CAD build for the part. Positions are in the model's coordinates, mm. A direction names the side the tool comes from. Give positions to 0.01 mm unless a question says otherwise; leave off trailing zeros. Order: outer loops, then holes, each group sorted by start corner. A loop starts at its lowest first (then second) coordinate and runs counter-clockwise, first axis right, second up.
Item 1: Two-plate mould, pull along Y, no slides. Class faces 5 (the flat face through (-11.45, -11.67, 10.4)), 6 (the cylindrical face through (0.605, -10.48, 0.989)), 7 (the flat face through (-11.17, 12.13, 0.96)): released by +Y, released by -Y, zero draft, split by the parting line, or undercut.
Item 2: Flat gauge pins, fed straight in: P1, Ø7.5, axis at y = -3.5, z = 10.5, coming from the +X side; P2, Ø0.9, axis at x = 11.5, y = 17, coming from the -Z side; P3, Ø6, axis at x = -9, z = 3, coming from the +Y side; P4, Ø6, axis at y = -4, z = 11, coming from the -X side. Where does each tip first touch, or does it go through?
Item 3: Wall check: L1, parallel to X at y = 7, z = 14; L2, parallel to X at y = 10, z = 9.25; L3, parallel to Y at x = 3, z = 1. Give the ranges that are in metal, low to high.
Item 4: Which spindle directions (+Z, -Z, +X, -X, +Y, -Y) get a long thin tool onto all of the face, cutting with end or side? Do faces 1 (the flat face through (-12.07, 7, 8)), 2 (the flat face through (0, -8, 1.95)), 3 (the cylindrical face through (-0.143, 5.981, 1.394)), 4 (the flat face through (-4, -15.948, 1)). Say none if no direction does.
Item 5: Band-saw the part on A-A on z = 2.5. Give the cut face in (x, y).
Item 6: Band-saw the part on B-B on x = -4. Give the cut face in (y, z).
Item 7: Band-saw the part on C-C on y = -2. Give the cut face in (x, z), plus the area to 3 significant figures.
Item 8: Band-saw the part on D-D on z = 11.5. Give the cut face in (x, y), plus the area to 3 significant figures.
```python
from build123d import *

# Parameters (mm, degrees)
BOSS_EXTRUDE1_DEPTH = 3.67
SKETCH2_W           = 3.67
SKETCH2_H           = 9.687937517
BOSS_EXTRUDE2_DEPTH = 9.735
SKETCH3_W           = 3.67
SKETCH3_H           = 26.515
BOSS_EXTRUDE3_DEPTH = 5.622062483
BOSS_EXTRUDE4_DEPTH = 20.5
SKETCH5_W           = 3.67
SKETCH5_H           = 15.31
BOSS_EXTRUDE5_DEPTH = 13.38
BOSS_EXTRUDE6_DEPTH = 2.35
SKETCH7_W           = 1.85
SKETCH7_H           = 17.78
CUT_EXTRUDE1_DEPTH  = 16.310000003
CUT_EXTRUDE2_REACH  = 27.99
SKETCH9_W           = 1.85
SKETCH9_H           = 17.78
CUT_EXTRUDE3_DEPTH  = 16.310000003
CUT_EXTRUDE4_REACH  = 26.67
CUT_EXTRUDE5_REACH  = 26.67
CUT_EXTRUDE6_DEPTH  = 26.99
CUT_EXTRUDE7_DEPTH  = 2.95
SKETCH15_W          = 1.68
SKETCH15_H          = 2.795
SKETCH16_W          = 1.68
SKETCH16_H          = 2.795
FILLET1_R           = 0.2
CUT_EXTRUDE8_DEPTH  = 1.31


with BuildPart() as part:
    # Sketch1 → Boss-Extrude1 (new body)
    with BuildSketch(Plane(origin=(-13.92, 0, 0), x_dir=(0, -1, 0), z_dir=(-1, 0, 0))):
        Polygon((19.9475, 5.622062483), (3.1675, 15.31), (3.1675, 5.622062483), align=None)
    extrude(amount=-BOSS_EXTRUDE1_DEPTH)

    # Sketch2 → Boss-Extrude2 (add)
    with BuildSketch(Plane(origin=(0, -3.1675, 0), x_dir=(-1, 0, 0), z_dir=(0, 1, 0))):
        with Locations((12.085, 10.466031242)):
            Rectangle(SKETCH2_W, SKETCH2_H)
    extrude(amount=BOSS_EXTRUDE2_DEPTH)

    # Sketch3 → Boss-Extrude3 (add)
    with BuildSketch(Plane(origin=(0, 0, 5.622062483), x_dir=(-1, 0, 0), z_dir=(0, 0, -1))):
        with Locations((12.085, -6.69)):
            Rectangle(SKETCH3_W, SKETCH3_H)
    extrude(amount=BOSS_EXTRUDE3_DEPTH)

    # Sketch4 → Boss-Extrude4 (add)
    with BuildSketch(Plane(origin=(-10.25, 0, 0), x_dir=(0, 0, -1), z_dir=(1, 0, 0))):
        with BuildLine():
            Line((3e-09, -19.9475), (-1.949999997, -19.9475))
            Line((-1.949999997, -19.9475), (-1.949999997, 4.6175))
            ThreePointArc((-1.949999997, 4.6175), (-1.37885822, 5.996358223), (3e-09, 6.5675))
            Line((3e-09, 6.5675), (3e-09, -19.9475))
        make_face()
    extrude(amount=BOSS_EXTRUDE4_DEPTH)

    # Sketch5 → Boss-Extrude5 (add)
    with BuildSketch(Plane(origin=(0, 6.5675, 0), x_dir=(-1, 0, 0), z_dir=(0, 1, 0))):
        with Locations((12.085, 7.655)):
            Rectangle(SKETCH5_W, SKETCH5_H)
    extrude(amount=BOSS_EXTRUDE5_DEPTH)

    # Sketch6 → Boss-Extrude6 (add)
    with BuildSketch(Plane(origin=(10.25, 0, 0), x_dir=(0, 0, -1), z_dir=(1, 0, 0))):
        Polygon((-15.31, -3.1675), (-15.31, 19.9475), (2e-09, 19.9475), (2e-09, -19.947499999), (-5.622062484, -19.947499999), align=None)
    extrude(amount=BOSS_EXTRUDE6_DEPTH)

    # Sketch7 → Cut-Extrude1 (cut, through all)
    with BuildSketch(Plane.XY.offset(15.31)):
        with Locations((12.995, 11.0575)):
            Rectangle(SKETCH7_W, SKETCH7_H)
    extrude(amount=-CUT_EXTRUDE1_DEPTH, mode=Mode.SUBTRACT)

    # Sketch8 → Cut-Extrude2 (cut, up to next)
    with BuildSketch(Plane(origin=(12.07, 0, 0), x_dir=(0, 0, -1), z_dir=(1, 0, 0)), mode=Mode.PRIVATE) as cut_extrude2_sk1:
        with BuildLine():
            Line((-8.04306505, 17.864239052), (-5.959804102, 19.9475))
            Line((-5.959804102, 19.9475), (-15.31, 19.9475))
            Line((-15.31, 19.9475), (-15.31, 10.26298277))
            ThreePointArc((-15.31, 10.26298277), (-13.200981436, 15.521010933), (-8.04306505, 17.864239052))
        make_face()
    cut_extrude2_tool1 = extrude(cut_extrude2_sk1.sketch, amount=-CUT_EXTRUDE2_REACH, mode=Mode.PRIVATE) & part.part
    add(cut_extrude2_tool1.solids().sort_by_distance((12.07, 17.788809, 12.169828))[0], mode=Mode.SUBTRACT)

    # Sketch9 → Cut-Extrude3 (cut, through all)
    with BuildSketch(Plane.XY.offset(15.31)):
        with Locations((-12.995, 11.0575)):
            Rectangle(SKETCH9_W, SKETCH9_H)
    extrude(amount=-CUT_EXTRUDE3_DEPTH, mode=Mode.SUBTRACT)

    # Sketch10 → Cut-Extrude4 (cut, up to next)
    with BuildSketch(Plane.ZY.offset(12.07), mode=Mode.PRIVATE) as cut_extrude4_sk1:
        Polygon((1.95, 13.1175), (1.95, 19.9475), (0, 19.9475), (0, 11.1675), align=None)
    cut_extrude4_tool1 = extrude(cut_extrude4_sk1.sketch, amount=-CUT_EXTRUDE4_REACH, mode=Mode.PRIVATE) & part.part
    add(cut_extrude4_tool1.solids().sort_by_distance((-12.07, 16.024701, 0.934401))[0], mode=Mode.SUBTRACT)

    # Sketch11 → Cut-Extrude5 (cut, up to next)
    with BuildSketch(Plane.ZY.offset(12.07), mode=Mode.PRIVATE) as cut_extrude5_sk1:
        with BuildLine():
            Line((5.959804102, 19.9475), (8.04306505, 17.864239052))
            ThreePointArc((8.04306505, 17.864239052), (13.200981436, 15.521010933), (15.31, 10.26298277))
            Line((15.31, 10.26298277), (15.31, 19.9475))
            Line((15.31, 19.9475), (5.959804102, 19.9475))
        make_face()
    cut_extrude5_tool1 = extrude(cut_extrude5_sk1.sketch, amount=-CUT_EXTRUDE5_REACH, mode=Mode.PRIVATE) & part.part
    add(cut_extrude5_tool1.solids().sort_by_distance((-12.07, 17.788809, 12.169828))[0], mode=Mode.SUBTRACT)

    # Sketch12 → Cut-Extrude6 (cut, through all)
    with BuildSketch(Plane(origin=(12.07, 0, 0), x_dir=(0, 0, -1), z_dir=(1, 0, 0))):
        Polygon((-1.95, 19.9475), (-1.95, 13.1175), (0, 11.1675), (0, 19.9475), align=None)
    extrude(amount=-CUT_EXTRUDE6_DEPTH, mode=Mode.SUBTRACT)

    # Sketch13 → Cut-Extrude7 (cut, through all)
    with BuildSketch(Plane.XY.offset(1.949999997)):
        with BuildLine():
            Line((-6.395488685, -12.9475), (-2.104511315, -12.9475))
            ThreePointArc((-2.104511315, -12.9475), (-0.604511315, -14.4475), (-2.104511315, -15.9475))
            Line((-2.104511315, -15.9475), (-6.395488685, -15.9475))
            ThreePointArc((-6.395488685, -15.9475), (-7.895488685, -14.4475), (-6.395488685, -12.9475))
        make_face()
        with BuildLine():
            Line((2.104511315, -8.947499999), (6.395488685, -8.947499999))
            ThreePointArc((6.395488685, -8.947499999), (7.895488685, -10.447499999), (6.395488685, -11.947499999))
            Line((6.395488685, -11.947499999), (2.104511315, -11.947499999))
            ThreePointArc((2.104511315, -11.947499999), (0.604511315, -10.447499999), (2.104511315, -8.947499999))
        make_face()
    extrude(amount=-CUT_EXTRUDE7_DEPTH, mode=Mode.SUBTRACT)

    # Sketch15 → Revolve1 (revolve)
    with BuildSketch(Plane.XY.offset(7.655)):
        with Locations((12.91, 11.61)):
            Rectangle(SKETCH15_W, SKETCH15_H)
    revolve(axis=Axis((12.07, 10.2125, 7.655), (1, 0, 0)))

    # Sketch16 → Revolve2 (revolve)
    with BuildSketch(Plane.XY.offset(7.655)):
        with Locations((-12.91, 11.61)):
            Rectangle(SKETCH16_W, SKETCH16_H)
    revolve(axis=Axis((-13.75, 10.2125, 7.655), (1, 0, 0)))

    # Fillet1
    fillet1_edges = [part.edges().sort_by_distance(p)[0] for p in [
        (13.75, 7.4175, 7.655),
        (-13.75, 7.4175, 7.655),
    ]]
    fillet(fillet1_edges, radius=FILLET1_R)

    # Sketch17 → Cut-Extrude8 (cut)
    with BuildSketch(Plane(origin=(-13.92, -19.9475, 5.622062483), x_dir=(0, 0, 1), z_dir=(-1, 0, 0))):
        Polygon((9.687937517, 22.115), (-5.622062486, 22.115), (-5.622062483, 0), (0, 0), (9.687937517, 16.78), align=None)
    extrude(amount=-CUT_EXTRUDE8_DEPTH, mode=Mode.SUBTRACT)


solid = part.part
```
The answers:
1. face 5: released by -Y
1. face 6: undercut
1. face 7: released by +Y
2. P1: stops at x = 12.6
2. P2: stops at z = 1.95
2. P3: stops at y = 19.95
2. P4: stops at x = -12.61
3. L1: x = -12.07 to -10.25, 10.25 to 12.07
3. L2: x = -13.75 to -10.25, 10.25 to 13.75
3. L3: y = -19.95 to -11.95, -8.95 to 6.29
4. face 1: -X
4. face 2: +Z, +Y, -Y
4. face 3: +Z, +Y
4. face 4: +Z, -Z
5. outline: (-12.61, -19.95) - (-10.25, -19.95) - (-10.25, 19.95) - (-12.07, 19.95) - (-12.07, 2.17) - (-12.61, 2.17) - close; (10.25, -19.95) - (12.6, -19.95) - (12.6, 2.17) - (12.07, 2.17) - (12.07, 19.95) - (10.25, 19.95) - close
6. outline: (-19.95, 0) - (-15.95, 0) - (-15.95, 1.95) - (-19.95, 1.95) - close; (-12.95, 0) - (6.57, 0) arc R1.95 ccw to (4.62, 1.95) - (-12.95, 1.95) - close
7. outline: (-12.61, 0) - (12.6, 0) - (12.6, 15.31) - (10.25, 15.31) - (10.25, 1.95) - (-10.25, 1.95) - (-10.25, 15.31) - (-12.61, 15.31) - close
7. area: 112 mm2
8. outline: (-12.61, -9.77) - (-10.25, -9.77) - (-10.25, 16.86) - (-12.07, 16.86) - (-12.07, 2.17) - (-12.61, 2.17) - close; (10.25, -9.77) - (12.6, -9.77) - (12.6, 2.17) - (12.07, 2.17) - (12.07, 16.86) - (10.25, 16.86) - close
8. area: 110 mm2
